Autodesk Inventor part; units mm, degrees
ref_plane "YZ Plane" through (0, 0, 0) normal (1, 0, 0) x (0, 1, 0)
ref_plane "XZ Plane" through (0, 0, 0) normal (0, 1, 0) x (-1, 0, 0)
ref_plane "XY Plane" through (0, 0, 0) normal (0, 0, 1) x (1, 0, 0)
sketch "Sketch1" plane through (0, 0, 0) normal (0, 1, 0) x (-1, 0, 0)
  line L0 (4, 4) -> (-6, 4)
  line L1 (-6, 4) -> (-6, -21)
  line L2 (-6, -21) -> (4, -21)
  line L3 (4, -21) -> (4, 4)
  point P0 (0, 0)
  dimension "d0" = 10
  dimension "d1" = 25
extrude "Extrusion1" add sketch "Sketch1" along normal blind 30
sketch "Sketch2" plane through (0, 30, 0) normal (0, 1, 0) x (1, 0, 0)
  line L0 (1, 28) -> (1, -15) construction
  line L1 (-4, 21) -> (-4, -4)
  circle A0 centre (1, 17) radius 2
  circle A1 centre (1, 0) radius 2
  line L2 (-4, -4) -> (6, -4)
  point P0 (0, 0)
  dimension "d5" = 5
  dimension "d6" = 4
  dimension "d7" = 4
  dimension "d8" = 17
  dimension "d9" = 4
  dimension "d10" = 25
hole "Hole1" at (1, 30, 0) at (1, 30, -17) direction (0, -1, 0) diameter 4 end through all
equation "\"d9\" = -0.5 * d8 + 0.5 * d10"
properties part number "mocowanie uchwytu02"
Geometry: final body of the model. Coordinates: model frame, mm. Round coordinates to 2 decimals unless told otherwise and drop trailing zeros. Loops run counter-clockwise (first coordinate to the right, second up) from the corner with the lowest first, then second, coordinate; pieces in that order, holes last.
Item 1: Section A-A, the plane x = 1. Output: boundary loops of the cut face in (y, z), plus the area to 3 significant figures.
Checked values:
outline: (0, -21) - (30, -21) - (30, -19) - (0, -19) - close; (0, -15) - (30, -15) - (30, -2) - (0, -2) - close; (0, 2) - (30, 2) - (30, 4) - (0, 4) - close
area: 510 mm2
Item 2: Contact query for flat-ended pins moving along their axis: P1, Ø6, axis at x = -0.5, z = 0, coming from the +Y side; P2, Ø3.5, axis at x = 1, z = 0, coming from the -Y side. Output: stop coordinate, or through.
Checked values:
P1: stops at y = 30
P2: passes through
Item 3: Line query: L1, parallel to Z at x = 1, y = 15.5; L2, parallel to X at y = 7.75, z = 0; L3, parallel to Z at x = -0.5, y = 4.75. Output: solid intervals per line, ascending.
Checked values:
L1: z = -21 to -19, -15 to -2, 2 to 4
L2: x = -4 to -1, 3 to 6
L3: z = -21 to -18.32, -15.68 to -1.32, 1.32 to 4
Item 4: Section C-C, the plane y = 15.5. Output: boundary loops of the cut face in (x, z), plus the area to 3 significant figures.
Checked values:
outline: (-4, -21) - (6, -21) - (6, 4) - (-4, 4) - close; hole circle Ø4 at (1, -17); hole circle Ø4 at (1, 0)
area: 225 mm2
Item 5: Section B-B, the plane z = -17. Output: boundary loops of the cut face in (x, y), plus the area to 3 significant figures.
Checked values:
outline: (-4, 0) - (-1, 0) - (-1, 30) - (-4, 30) - close; (3, 0) - (6, 0) - (6, 30) - (3, 30) - close
area: 180 mm2
Item 6: Mould query, pull axis Z, two halves, no side actions, for faces 1 (the flat face through (6, 15, -8)), 2 (the flat face through (1, 15, -21)), 3 (the cylindrical face through (0.399, 14.79, 1.908)). Classes: released by +Z, released by -Z, zero draft, split by the parting line, or undercut.
Checked values:
face 1: zero draft
face 2: released by -Z
face 3: undercut
Item 7: Section D-D, the plane z = -1. Output: boundary loops of the cut face in (x, y), plus the area to 3 significant figures.
Checked values:
outline: (-4, 0) - (-0.73, 0) - (-0.73, 30) - (-4, 30) - close; (2.73, 0) - (6, 0) - (6, 30) - (2.73, 30) - close
area: 196 mm2
